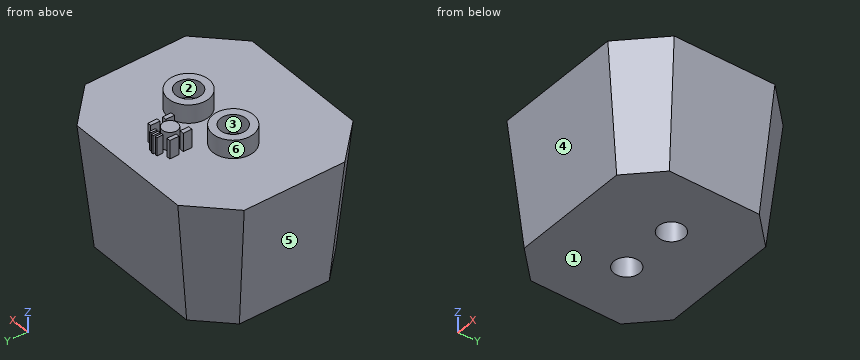
```python
from build123d import *

# Parameters (mm, degrees)
SKETCH1_R           = 12.5
BOSS_EXTRUDE1_DEPTH = 122
BOSS_EXTRUDE1_DRAFT = -6
SKETCH2_R           = 19.8
SKETCH2_R_2         = 12.5
SKETCH2_R_3         = 7.5
SKETCH2_W           = 2
SKETCH2_H           = 6
SKETCH2_H_2         = 6.8
SKETCH2_W_2         = 3.6
SKETCH2_H_3         = 9
SKETCH2_W_3         = 4
SKETCH2_H_4         = 8.4
BOSS_EXTRUDE2_DEPTH = 140


with BuildPart() as part:
    # Sketch1 → Boss-Extrude1 (with draft: the straight prism first)
    with BuildSketch(Plane.XY):
        Polygon((-58, 73), (-87, 44), (-87, -44), (-58, -73), (58, -73), (87, -44), (87, 44), (58, 73), align=None)
        with Locations((-28, 4)):
            Circle(SKETCH1_R, mode=Mode.SUBTRACT)
        with Locations((28, 4)):
            Circle(SKETCH1_R, mode=Mode.SUBTRACT)
    extrude(amount=BOSS_EXTRUDE1_DEPTH)
    # Boss-Extrude1: the draft: its side faces are tilted about the plane it starts from
    boss_extrude1_sides = [part.faces().sort_by_distance(p)[0] for p in [
        (-72.5, 58.5, 61),
        (-87, 0, 61),
        (-72.5, -58.5, 61),
        (0, -73, 61),
        (72.5, -58.5, 61),
        (87, 0, 61),
        (72.5, 58.5, 61),
        (0, 73, 61),
        (-40.5, 4, 61),
        (15.5, 4, 61),
    ]]
    draft(boss_extrude1_sides, Plane.XY, BOSS_EXTRUDE1_DRAFT)

    # Sketch2 → Boss-Extrude2 (add)
    # profile 1 of 10: a face of its own
    with BuildSketch(Plane.XY):
        with Locations(Location((-28, 4, 0), (0, 0, 180))):
            Circle(SKETCH2_R)
        with Locations(Location((-28, 4, 0), (0, 0, 180))):
            Circle(SKETCH2_R_2, mode=Mode.SUBTRACT)
    # profile 2 of 10: a face of its own
    with BuildSketch(Plane.XY):
        with Locations(Location((28, 4, 0), (0, 0, 180))):
            Circle(SKETCH2_R)
        with Locations(Location((28, 4, 0), (0, 0, 180))):
            Circle(SKETCH2_R_2, mode=Mode.SUBTRACT)
    # profile 3 of 10: a face of its own
    with BuildSketch(Plane.XY):
        with Locations(Location((0, 44, 0), (0, 0, 180))):
            Circle(SKETCH2_R_3)
    # profile 4 of 10: a face of its own
    with BuildSketch(Plane.XY):
        with Locations((-3.8, 57.5)):
            Rectangle(SKETCH2_W, SKETCH2_H)
    # profile 5 of 10: a face of its own
    with BuildSketch(Plane.XY):
        with Locations((0, 58)):
            Rectangle(SKETCH2_W, SKETCH2_H_2)
    # profile 6 of 10: a face of its own
    with BuildSketch(Plane.XY):
        with Locations((3.8, 57.5)):
            Rectangle(SKETCH2_W, SKETCH2_H)
    # profile 7 of 10: a face of its own
    with BuildSketch(Plane.XY):
        with Locations((-12, 50.5)):
            Rectangle(SKETCH2_W_2, SKETCH2_H_3)
    # profile 8 of 10: a face of its own
    with BuildSketch(Plane.XY):
        with Locations((12, 50.5)):
            Rectangle(SKETCH2_W_2, SKETCH2_H_3)
    # profile 9 of 10: a face of its own
    with BuildSketch(Plane.XY):
        with Locations((-11, 37)):
            Rectangle(SKETCH2_W_3, SKETCH2_H_4)
    # profile 10 of 10: a face of its own
    with BuildSketch(Plane.XY):
        with Locations((11, 37)):
            Rectangle(SKETCH2_W_3, SKETCH2_H_4)
    extrude(amount=BOSS_EXTRUDE2_DEPTH)


solid = part.part
```
Verification items for the finished model (mm, model axes). Face numbers are marked on the shaded views. A direction names the side the tool comes from. Round coordinates to 2 decimals unless told otherwise and drop trailing zeros. Order: outer loops, then holes, each group sorted by start corner. A loop starts at its lowest first (then second) coordinate and runs counter-clockwise, first axis right, second up. Notation, with made-up numbers: (16.25, 18) -> (43.25, 18) arc R9 ccw to (43.25, 24) -> close; hole circle Ø9 at (-22, -20). An arc over 180 degrees is marked (long way). Put each result on its own line as item: value. Start each with the question number.
(1) Tool access check on the marked faces 5 and 6. Record the directions out of +Z, -Z, +X, -X, +Y, -Y that give a thin tool (end or side, any length) a straight path to the whole face; none if there is none.
(2) Section check A-A (z = 131). State how many separate pieces and enclosed holes the cut face has, then the cut area to 3 significant figures.
(3) Material ranges on line 1 along Y through (x, z) = (-28, 131.5); line 2 along Z through (x, y) = (-71.5, -59); line 3 along X through (y, z) = (67, 105.5), recorded low to high.
(4) Section check C-C (z = 14). Enter the section's corners in (x, y).
(5) Depth check by flat-ended pin: pin 1 Ø9 at (y, z) = (36, 127) entering from +X; pin 2 Ø4.5 at (x, z) = (10.5, 129) entering from -Y; pin 3 Ø6 at (x, z) = (-42.5, 26) entering from -Y. Enter the tip coordinate at first touch or a pass-through.
(6) Section check B-B (x = -44). Enter the section's corners in (y, z).
(7) Draft check along Y on the marked faces 1, 2, 3 and 4. Enter one of: +Y half, -Y half, draft (parallel to the pull), parting line (faces both ways), or undercut.
(8) Section check D-D (z = 98.5). Enter the section's corners in (x, y), then the cut area to 3 significant figures.
Completed:
1. face 5: -Z, -X, +Y, -Y
1. face 6: +Z
2. separate pieces: 10
2. enclosed holes: 2
2. area: 1,830 mm2
3. line 1: y = -15.8 to -8.5, 16.5 to 23.8
3. line 2: z = 0 to 122
3. line 3: x = -79.68 to 79.68
4. outline: (-88.47, -44.61) -> (-58.61, -74.47) -> (58.61, -74.47) -> (88.47, -44.61) -> (88.47, 44.61) -> (58.61, 74.47) -> (-58.61, 74.47) -> (-88.47, 44.61) -> close; hole circle Ø22.06 at (-28, 4); hole circle Ø22.06 at (28, 4)
5. pin 1: stops at x = 13
5. pin 2: stops at y = -8.63
5. pin 3: stops at y = -76.05
6. outline: (-85.82, 122) -> (-73, 0) -> (73, 0) -> (85.82, 122) -> (15.66, 122) -> (15.66, 140) -> (-7.66, 140) -> (-7.66, 122) -> close
7. face 1: draft
7. face 2: undercut
7. face 3: undercut
7. face 4: -Y half
8. outline: (-97.35, -48.29) -> (-62.29, -83.35) -> (62.29, -83.35) -> (97.35, -48.29) -> (97.35, 48.29) -> (62.29, 83.35) -> (-62.29, 83.35) -> (-97.35, 48.29) -> close; hole circle Ø4.29 at (-28, 4); hole circle Ø4.29 at (28, 4)
8. area: 30,000 mm2
